Here's how the part is built. I have some questions about the finished solid (model axes, mm). A direction names the side the tool comes from. Give positions to 0.01 mm unless a question says otherwise; leave off trailing zeros. Loops run counter-clockwise (first coordinate to the right, second up) from the corner with the lowest first, then second, coordinate; pieces in that order, holes last. Notation, with made-up numbers: (59, 76) - (88, 76) arc R28 cw to (88, 113) - close; hole circle Ø5 at (76.5, 13). An arc over 180 degrees is marked (long way). Return JSON: item names as keys, results as strings. Group by question number.
(1) If we section it at C-C (y = 10.5): Please give me the cut outline in (x, z), then the cut area to 3 significant figures.
(2) If we section it at A-A (x = 0): State how many separate pieces and enclosed holes the cut face has, then the cut area to 3 significant figures.
(3) If we mould it in two halves opening along Z, with no side actions, what happens to faces 5 (the flat face through (17.45, -1, -12)), 6 (the cylindrical face through (-0.075, 17.994, 3.454)), 7 (the conical face through (18.16, 0.98, 1.83)), 8 (the conical face through (-0.08, -21.51, 1.83))? For each: released by +Z, released by -Z, zero draft, split by the parting line, or undercut.
(4) I need wall thicknesses on probe 1 along Y at (x, z) = (-6, 1); probe 2 along X at (y, z) = (4, -18); probe 3 along Y at (x, z) = (-1, -17). Which ranges of each line are inside material? Lowest first, please. Write a range as [from, to].
(5) On a 3-axis mill with a long thin cutter (end or side, diameter ignored), from which of +Z, -Z, +X, -X, +Y, -Y can I reach the whole of each face in a straight line? I mean faces 1 (the flat face through (8.15, -0.22, -25.398)), 2 (the flat face through (7.95, 0, -27)), 3 (the flat face through (4.95, -1, 3)), 4 (the flat face through (-7, 5.5, -14)). Say none if no direction works.
(6) If we section it at D-D (x = 9): Please give me the cut outline in (y, z), then the cut area to 3 significant figures.
(7) For P1, Ø1, axis at x = 5, y = -16, coming from the -Z side; P2, Ø10, axis at y = -1.5, z = -18, coming from the -X side; P3, Ø1, axis at x = 8.5, z = -9, coming from the +Y side, each with a flat end and sliding along its axis, tell me the tip position at first contact or that it passes through.
```python
from build123d import *

# Parameters (mm, degrees)
SKETCH1_R                                      = 29.692527183
SKETCH1_R_2                                    = 22.692527183
SKETCH1_R_3                                    = 19.692527183
SKETCH1_R_4                                    = 16.692527183
BOSS_EXTRUDE1_DEPTH                            = 5
SKETCH9_W                                      = 27.5
SKETCH9_H                                      = 28
BOSS_EXTRUDE2_DEPTH                            = 7.5
SKETCH10_W                                     = 23.5
SKETCH10_H                                     = 25.45
CUT_EXTRUDE1_DEPTH                             = 6.1
SKETCH12_W                                     = 12
SKETCH12_H                                     = 11
CUT_EXTRUDE2_DEPTH                             = 3
SKETCH11_W                                     = 13
SKETCH11_H                                     = 9.717675131
CUT_EXTRUDE3_DEPTH                             = 4.947760199
CSK_FOR_M3_FLAT_HEAD_MACHINE_SCREW1_AT_2_COUNT = 2
CSK_FOR_M3_FLAT_HEAD_MACHINE_SCREW1_AT_2_PITCH = 27.84943902
CSK_FOR_M3_FLAT_HEAD_MACHINE_SCREW1_AT_3_COUNT = 2
CSK_FOR_M3_FLAT_HEAD_MACHINE_SCREW1_AT_3_PITCH = 27.84943902
CSK_FOR_M3_FLAT_HEAD_MACHINE_SCREW1_AT_4_COUNT = 2
CSK_FOR_M3_FLAT_HEAD_MACHINE_SCREW1_AT_4_PITCH = 39.385054366
SPLIT1_START                                   = 5.5
SPLIT1_OUTLINE_W                               = 27.5
SPLIT1_OUTLINE_H                               = 28
SPLIT1_DEPTH                                   = 2
SPLIT1_START_2                                 = -28
SPLIT1_2_DEPTH                                 = 28
SPLIT1_3_OUTLINE_W                             = 23.5
SPLIT1_3_OUTLINE_H                             = 0.6
SPLIT1_3_DEPTH                                 = 2.602239801


# Read off the part's stored shape, not the designer's step: Split1
with BuildPart() as part:
    # Sketch1 → Boss-Extrude1 (new body)
    # profile 1 of 4: a face of its own
    with BuildSketch(Plane(origin=(0, 0, 0), x_dir=(-1, 0, 0), z_dir=(0, 0, 1))):
        with Locations(Location((0, 0, 0), (0, 0, 180))):
            Circle(SKETCH1_R)
        Circle(SKETCH1_R_2, mode=Mode.SUBTRACT)
    # profile 2 of 4: a face of its own
    with BuildSketch(Plane(origin=(0, 0, 0), x_dir=(-1, 0, 0), z_dir=(0, 0, 1))):
        Circle(SKETCH1_R_2)
        Circle(SKETCH1_R_3, mode=Mode.SUBTRACT)
    # profile 3 of 4: a face of its own
    with BuildSketch(Plane(origin=(0, 0, 0), x_dir=(-1, 0, 0), z_dir=(0, 0, 1))):
        Circle(SKETCH1_R_3)
        Circle(SKETCH1_R_4, mode=Mode.SUBTRACT)
    # profile 4 of 4: a face of its own
    with BuildSketch(Plane(origin=(0, 0, 0), x_dir=(-1, 0, 0), z_dir=(0, 0, 1))):
        with BuildLine():
            Line((14.058465911, 9), (-14.058465911, 9))
            ThreePointArc((-14.058465911, 9), (-16.692527183, 0), (-14.058465911, -9))
            Line((-14.058465911, -9), (14.058465911, -9))
            ThreePointArc((14.058465911, -9), (16.020483578, -4.688770595), (16.692527183, 0))
            ThreePointArc((16.692527183, 0), (16.020483578, 4.688770595), (14.058465911, 9))
        make_face()
    extrude(amount=BOSS_EXTRUDE1_DEPTH)

    # Sketch9 → Boss-Extrude2 (add, symmetric)
    with BuildSketch(Plane(origin=(0, 0, 0), x_dir=(1, 0, 0), z_dir=(0, 1, 0))):
        with Locations((5.7, 14)):
            Rectangle(SKETCH9_W, SKETCH9_H)
    extrude(amount=BOSS_EXTRUDE2_DEPTH, both=True)

    # Sketch10 → Cut-Extrude1 (cut, symmetric)
    with BuildSketch(Plane(origin=(0, 0, 0), x_dir=(1, 0, 0), z_dir=(0, 1, 0))):
        with Locations((5.7, 12.672760199)):
            Rectangle(SKETCH10_W, SKETCH10_H)
    extrude(amount=CUT_EXTRUDE1_DEPTH, both=True, mode=Mode.SUBTRACT)

    # Sketch12 → Cut-Extrude2 (cut)
    with BuildSketch(Plane.XY.offset(-28)):
        with Locations((1.95, 0)):
            Rectangle(SKETCH12_W, SKETCH12_H)
    extrude(amount=CUT_EXTRUDE2_DEPTH, mode=Mode.SUBTRACT)

    # Sketch11 → Cut-Extrude3 (cut)
    with BuildSketch(Plane.XY.offset(5)):
        with Locations((-1.55, -0.433824782)):
            Rectangle(SKETCH11_W, SKETCH11_H)
    extrude(amount=-CUT_EXTRUDE3_DEPTH, mode=Mode.SUBTRACT)

    # Sketch13 → CSK for M3 Flat Head Machine Screw1 (revolve, cut)
    with BuildSketch(Plane.YZ.offset(-19.692527183)):
        Polygon((0, 0), (0, 13.021463052), (1.7, 12), (1.7, 1.95), (3.65, 0), align=None)
    csk_for_m3_flat_head_machine_screw1 = revolve(axis=Axis((-19.692527183, 0, -6.35), (0, 0, 1)), mode=Mode.SUBTRACT)

    # CSK for M3 Flat Head Machine Screw1 at 2: CSK for M3 Flat Head Machine Screw1 ×2
    with Locations(*[Vector(0.7071067811865476, -0.7071067811865475, 0) * (i * CSK_FOR_M3_FLAT_HEAD_MACHINE_SCREW1_AT_2_PITCH) for i in range(1, CSK_FOR_M3_FLAT_HEAD_MACHINE_SCREW1_AT_2_COUNT)]):
        add(csk_for_m3_flat_head_machine_screw1, mode=Mode.SUBTRACT)

    # CSK for M3 Flat Head Machine Screw1 at 3: CSK for M3 Flat Head Machine Screw1 ×2
    with Locations(*[Vector(0.7071067811865476, 0.7071067811865475, 0) * (i * CSK_FOR_M3_FLAT_HEAD_MACHINE_SCREW1_AT_3_PITCH) for i in range(1, CSK_FOR_M3_FLAT_HEAD_MACHINE_SCREW1_AT_3_COUNT)]):
        add(csk_for_m3_flat_head_machine_screw1, mode=Mode.SUBTRACT)

    # CSK for M3 Flat Head Machine Screw1 at 4: CSK for M3 Flat Head Machine Screw1 ×2
    with Locations(*[(i * CSK_FOR_M3_FLAT_HEAD_MACHINE_SCREW1_AT_4_PITCH, 0, 0) for i in range(1, CSK_FOR_M3_FLAT_HEAD_MACHINE_SCREW1_AT_4_COUNT)]):
        add(csk_for_m3_flat_head_machine_screw1, mode=Mode.SUBTRACT)

    # Split1 outline → Split1 (cut)
    with BuildSketch(Plane(origin=(0, 0, 0), x_dir=(1, 0, 0), z_dir=(0, 1, 0)).offset(SPLIT1_START)):
        with Locations((5.7, 14)):
            Rectangle(SPLIT1_OUTLINE_W, SPLIT1_OUTLINE_H)
    extrude(amount=SPLIT1_DEPTH, mode=Mode.SUBTRACT)


with BuildPart() as body_2:
    # Split1 2 outline → Split1 2 (new body)
    with BuildSketch(Plane.XY.offset(SPLIT1_START_2)):
        Polygon((-8.05, 5.5), (-6.05, 5.5), (-6.05, 6.1), (17.45, 6.1), (17.45, 5.5), (19.45, 5.5), (19.45, 7.5), (-8.05, 7.5), align=None)
    extrude(amount=SPLIT1_2_DEPTH)

    # Split1 3 outline → Split1 3 (add)
    with BuildSketch(Plane.XY.offset(SPLIT1_START_2)):
        with Locations((5.7, 5.8)):
            Rectangle(SPLIT1_3_OUTLINE_W, SPLIT1_3_OUTLINE_H)
    extrude(amount=SPLIT1_3_DEPTH)


solid = part.part
```
Values:
{
 "1": {"outline": "(-27.77, 0) - (-12.98, 0) - (-12.98, 5) - (-27.77, 5) - close; (12.98, 0) - (27.77, 0) - (27.77, 5) - (12.98, 5) - close", "area": "148 mm2"},
 "2": {"separate pieces": "6", "enclosed holes": "0", "area": "171 mm2"},
 "3": {"face 5": "undercut", "face 6": "zero draft", "face 7": "undercut", "face 8": "released by -Z"},
 "4": {"probe 1": "[-29.08, -15.58], [-9, -5.29], [4.43, 9], [15.58, 29.08]", "probe 2": "[-8.05, -6.05], [17.45, 19.45]", "probe 3": "[-7.5, -6.1]"},
 "5": {"face 1": "+Y", "face 2": "-Z, +Y", "face 3": "+Z, -Z", "face 4": "-Z, +X, -X, +Y"},
 "6": {"outline": "(-28.3, 0) - (-14.06, 0) - (-14.06, 5) - (-28.3, 5) - close; (-9, 0) - (-7.5, 0) - (-7.5, -28) - (5.5, -28) - (5.5, -25.4) - (-6.1, -25.4) - (-6.1, 0.05) - (6.1, 0.05) - (6.1, 0) - (9, 0) - (9, 5) - (-9, 5) - close; (14.06, 0) - (28.3, 0) - (28.3, 5) - (14.06, 5) - close", "area": "301 mm2"},
 "7": {"P1": "z = 0", "P2": "x = -8.05", "P3": "y = -6.1"}
}
